CAD build for the part. Positions are in the model's coordinates, mm. Coordinates: 2 decimals unless noted, no trailing zeros. Loops run counter-clockwise (first coordinate to the right, second up) from the corner with the lowest first, then second, coordinate; pieces in that order, holes last. Notation, with made-up numbers: (27.25, 14.5) -> (62.25, 14.5) arc R13 ccw to (62.25, 32.5) -> close; hole circle Ø2 at (70.5, 89). An arc over 180 degrees is marked (long way). Write item = value, one per line. Start each with the question number.
(1) Band-saw the part on C-C (y = 0.25). Count the separate pieces of the cut face and the enclosed holes in it, and give its area (3 significant figures).
(2) Drill centre lines: line 1 (Z direction, x = 44.5, y = 0.5); line 2 (Z direction, x = 24.5, y = 0.4); line 3 (X direction, y = 1.05, z = -13.5). Where is each one in solid material? Low to high. Write a range as from..to.
(3) Band-saw the part on B-B (z = -13.5). Write the cut outline in (x, y), and give its area (3 significant figures).
(4) Band-saw the part on D-D (x = 44.5). Write the cut outline in (y, z).
(5) Pull direction Z, two halves, no side cores. Call faces 1 (the face through (24, 1, -27)), 2 (the face through (43.39, 0.76, -23.51)), 3 (the face through (0, 1, -13)): +Z half, -Z half, draft (parallel to the pull), parting line (faces both ways), or undercut.
(6) Flat gauge pin, fed straight in: P1, Ø2.5, axis at x = 44.5, z = -4.5, coming from the -Y side. Where does the tip first touch, or does it go through?
(7) Band-saw the part on A-A (x = 34). Write the cut outline in (y, z).
```python
from build123d import *

# Parameters (mm, degrees)
SKETCH1_W               = 49
SKETCH1_H               = 27
BOSS_EXTRUDE1_DEPTH     = 1.5
SKETCH2_R               = 1.5
CUT_EXTRUDE1_DEPTH      = 10
CUT_EXTRUDE1_DEPTH_BACK = 10
SKETCH3_R               = 1.5
SKETCH3_R_2             = 4
CUT_EXTRUDE2_DEPTH      = 10
CUT_EXTRUDE2_DEPTH_BACK = 10


with BuildPart() as part:
    # Sketch1 → Boss-Extrude1 (new body)
    with BuildSketch(Plane(origin=(0, 0, 0), x_dir=(1, 0, 0), z_dir=(0, 1, 0))):
        with Locations((24.5, 13.5)):
            Rectangle(SKETCH1_W, SKETCH1_H)
    extrude(amount=BOSS_EXTRUDE1_DEPTH)

    # Sketch2 → Cut-Extrude1 (cut, two sides)
    with BuildSketch(Plane(origin=(0, 1.5, 0), x_dir=(1, 0, 0), z_dir=(0, 1, 0))) as cut_extrude1_sk:
        with Locations((4.5, 22.5)):
            Circle(SKETCH2_R)
        with Locations((4.5, 4.5)):
            Circle(SKETCH2_R)
        with Locations((44.5, 4.5)):
            Circle(SKETCH2_R)
        with Locations((44.5, 22.5)):
            Circle(SKETCH2_R)
    extrude(amount=CUT_EXTRUDE1_DEPTH, mode=Mode.SUBTRACT)
    extrude(cut_extrude1_sk.sketch, amount=-CUT_EXTRUDE1_DEPTH_BACK, mode=Mode.SUBTRACT)

    # Sketch3 → Cut-Extrude2 (cut, two sides)
    with BuildSketch(Plane(origin=(0, 1.5, 0), x_dir=(1, 0, 0), z_dir=(0, 1, 0))) as cut_extrude2_sk:
        with Locations((15, 13.5)):
            Circle(SKETCH3_R)
        with Locations((34, 13.5)):
            Circle(SKETCH3_R)
        with Locations((24.5, 21.5)):
            Circle(SKETCH3_R)
        with Locations((24.5, 5.5)):
            Circle(SKETCH3_R)
        with Locations((24.5, 13.5)):
            Circle(SKETCH3_R_2)
    extrude(amount=CUT_EXTRUDE2_DEPTH, mode=Mode.SUBTRACT)
    extrude(cut_extrude2_sk.sketch, amount=-CUT_EXTRUDE2_DEPTH_BACK, mode=Mode.SUBTRACT)


solid = part.part
```
Findings below:
q1.separate_pieces = 1
q1.enclosed_holes = 9
q1.area = 1,220 mm²
q2.line_1 = -27..-24, -21..-6, -3..0
q2.line_2 = -27..-23, -20..-17.5, -9.5..-7, -4..0
q2.line_3 = 0..13.5, 16.5..20.5, 28.5..32.5, 35.5..49
q3.outline = (0, 0) -> (13.5, 0) -> (13.5, 1.5) -> (0, 1.5) -> close; (16.5, 0) -> (20.5, 0) -> (20.5, 1.5) -> (16.5, 1.5) -> close; (28.5, 0) -> (32.5, 0) -> (32.5, 1.5) -> (28.5, 1.5) -> close; (35.5, 0) -> (49, 0) -> (49, 1.5) -> (35.5, 1.5) -> close
q3.area = 52.5 mm²
q4.outline = (0, -27) -> (1.5, -27) -> (1.5, -24) -> (0, -24) -> close; (0, -21) -> (1.5, -21) -> (1.5, -6) -> (0, -6) -> close; (0, -3) -> (1.5, -3) -> (1.5, 0) -> (0, 0) -> close
q5.face_1 = -Z half
q5.face_2 = undercut
q5.face_3 = draft
q6.P1 = through
q7.outline = (0, -27) -> (1.5, -27) -> (1.5, -15) -> (0, -15) -> close; (0, -12) -> (1.5, -12) -> (1.5, 0) -> (0, 0) -> close
